Design review of the part built by this model. Coordinates are the model's own, in mm. A direction names the side the tool comes from. Give positions to 0.01 mm unless a question says otherwise; leave off trailing zeros. Write each loop counter-clockwise with the first axis right and the second up, starting at its lowest first coordinate (ties: lowest second). Pieces come first, ordered by that corner, then holes. Notation, with made-up numbers: M 57,87.5 L 115,87.5 A19 ccw 115,121.5 Z; hole C 75,27.25 d4. An arc over 180 degrees is marked long. Write each question's results on one line, items separated by ' | '. Start each with the question number.
from build123d import *

# Parameters (mm, degrees)
BOSS_EXTRUDE2_DEPTH     = 20
CUT_EXTRUDE2_DEPTH      = 42.231056256
CUT_EXTRUDE2_DEPTH_BACK = 42.231056256
SKETCH4_W               = 5
SKETCH4_H               = 25
CUT_EXTRUDE3_DEPTH      = 42.231056256
CUT_EXTRUDE3_DEPTH_BACK = 42.231056256
SKETCH5_R               = 1.25
BOSS_EXTRUDE3_DEPTH     = 20
CUT_EXTRUDE4_DEPTH      = 42.231056256
CUT_EXTRUDE4_DEPTH_BACK = 42.231056256
SKETCH7_R               = 1.25


with BuildPart() as part:
    # Sketch3 → Boss-Extrude2 (new body)
    with BuildSketch(Plane.XY):
        with BuildLine():
            Line((0, 0), (20, 0))
            Line((20, 0), (20, 20))
            ThreePointArc((20, 20), (10, 30), (0, 20))
            Line((0, 20), (0, 0))
        make_face()
    extrude(amount=BOSS_EXTRUDE2_DEPTH)

    # Sketch4 → Cut-Extrude2 (cut, two sides: drawn at the far end of the back side and taken through both)
    with BuildSketch(Plane(origin=(20, 0, 0), x_dir=(0, 0, -1), z_dir=(1, 0, 0)).offset(-CUT_EXTRUDE2_DEPTH_BACK)):
        with Locations((-10, 17.5)):
            Rectangle(SKETCH4_W, SKETCH4_H)
    extrude(amount=CUT_EXTRUDE2_DEPTH + CUT_EXTRUDE2_DEPTH_BACK, mode=Mode.SUBTRACT)

    # Sketch5 → Cut-Extrude3 (cut, two sides: drawn at the far end of the back side and taken through both)
    with BuildSketch(Plane(origin=(0, 0, 0), x_dir=(-1, 0, 0), z_dir=(0, 0, -1)).offset(-CUT_EXTRUDE3_DEPTH_BACK)):
        with Locations((-10, 20)):
            Circle(SKETCH5_R)
    extrude(amount=CUT_EXTRUDE3_DEPTH + CUT_EXTRUDE3_DEPTH_BACK, mode=Mode.SUBTRACT)

    # Sketch6 → Boss-Extrude3 (add)
    with BuildSketch(Plane(origin=(20, 0, 0), x_dir=(0, 0, -1), z_dir=(1, 0, 0))):
        with BuildLine():
            Line((-20, 0), (0, 0))
            ThreePointArc((0, 0), (-10, -10), (-20, 0))
        make_face()
    extrude(amount=-BOSS_EXTRUDE3_DEPTH)

    # Sketch7 → Cut-Extrude4 (cut, two sides: drawn at the far end of the back side and taken through both)
    with BuildSketch(Plane(origin=(20, 0, 0), x_dir=(0, 0, -1), z_dir=(1, 0, 0)).offset(-CUT_EXTRUDE4_DEPTH_BACK)):
        with Locations((-10, 0)):
            Circle(SKETCH7_R)
    extrude(amount=CUT_EXTRUDE4_DEPTH + CUT_EXTRUDE4_DEPTH_BACK, mode=Mode.SUBTRACT)


solid = part.part
Q1. The part is to be moulded in two halves that separate along X. For faces 1 (the flat face through (0, 2, 10)), 2 (the flat face through (10, 17, 12.5)), 3 (the cylindrical face through (10.99, 19.24, 3.8)), say which applies: pulls with the +X half, pulls with the -X half, needs draft (parallel to the pull), parting line crosses it, or undercut.
Q2. We need section A-A on x = 10. Write out the cut boundary in (y, z), and give its area (3 significant figures).
Q3. For faces 4 (the flat face through (10, 15, 20)), 5 (the flat face through (10, 5, 10)), list the 3-axis set-ups (+Z, -Z, +X, -X, +Y, -Y) from which the entire face can be reached by the end or side of a thin tool; tool diameter is ignored.
Q4. We need section D-D on x = 6.75. Write out the cut boundary in (y, z).
Q5. Wall thickness on line 1 along Z through (x, y) = (16.25, 23.5); line 2 along Y through (x, z) = (9.25, 10); line 3 along X through (y, z) = (20, 3.5): over which ranges is each line inside the solid? List them lowest first. Write a range as from..to.
Q6. We need section B-B on z = 10. Write out the cut boundary in (x, y).
Q7. For pin 1 Ø4 at (x, z) = (9.5, 11) entering from +Y; pin 2 Ø2 at (y, z) = (0, 10) entering from -X; pin 3 Ø1.5 at (x, y) = (14.5, -5.5) entering from +Z; pin 4 Ø6 at (x, z) = (4.5, 6.5) entering from +Y, all flat-tipped, find the tip position at first contact; note any pin that passes through.
Q8. We need section C-C on y = 9. Write out the cut boundary in (x, z), and give its area (3 significant figures).
Answer sheet:
1) face 1: pulls with the -X half | face 2: needs draft | face 3: undercut
2) outline: M 0,0 L 18.75,0 L 18.75,7.5 L 5,7.5 L 5,12.5 L 18.75,12.5 L 18.75,20 L 0,20 A10 ccw Z; M 21.25,0 L 30,0 L 30,7.5 L 21.25,7.5 Z; M 21.25,12.5 L 30,12.5 L 30,20 L 21.25,20 Z; hole C 0,10 d2.5 | area: 590 mm^2
3) face 4: +Z, +X, -X, +Y, -Y | face 5: +X, -X, +Y
4) outline: M 0,0 L 29.46,0 L 29.46,7.5 L 5,7.5 L 5,12.5 L 29.46,12.5 L 29.46,20 L 0,20 A10 ccw Z; hole C 0,10 d2.5
5) line 1: 0..7.5, 12.5..20 | line 2: -10..-1.25, 1.25..5 | line 3: 0..8.75, 11.25..20
6) outline: M 0,-10 L 20,-10 L 20,-1.25 L 0,-1.25 Z; M 0,1.25 L 20,1.25 L 20,5 L 0,5 Z
7) pin 1: y = 30 | pin 2: through | pin 3: z = 18.8 | pin 4: y = 29.68
8) outline: M 0,0 L 20,0 L 20,7.5 L 0,7.5 Z; M 0,12.5 L 20,12.5 L 20,20 L 0,20 Z | area: 300 mm^2
